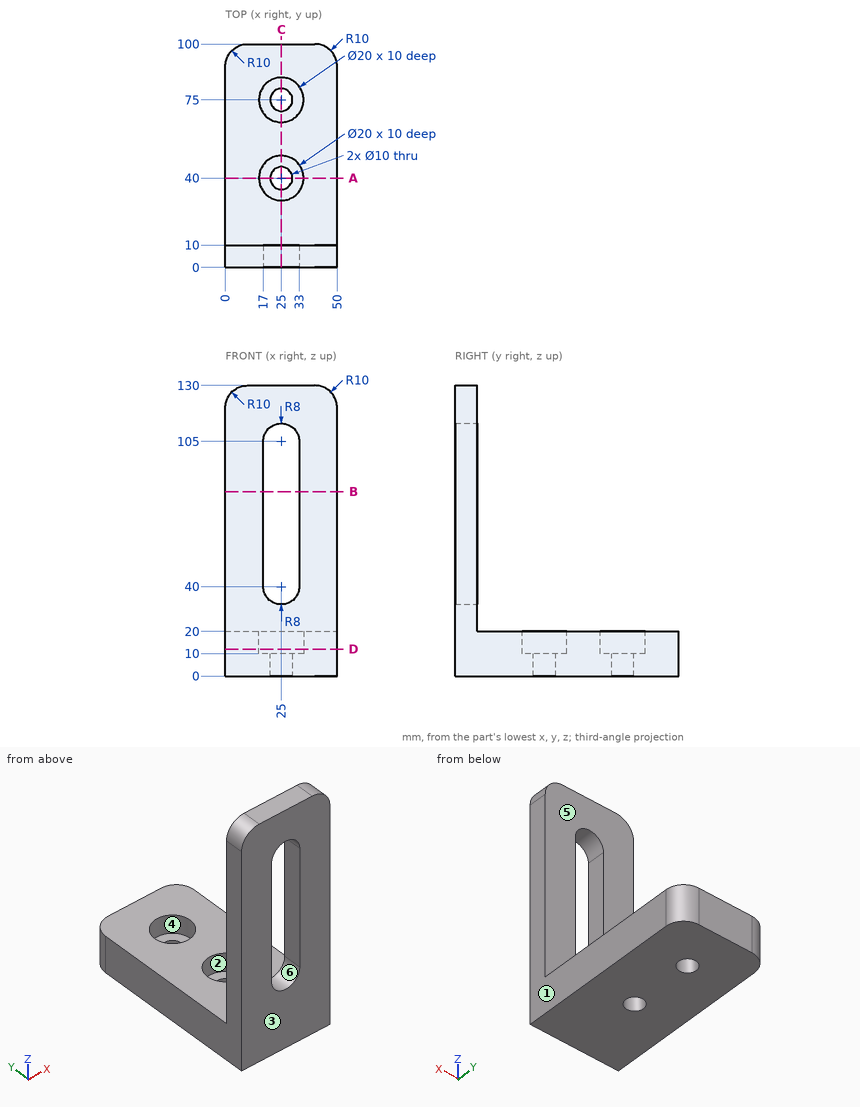
Can you work these out from the drawing? Everything is in mm from the part's minimum corner. A direction names the side the tool comes from. Coordinates: 2 decimals unless noted, no trailing zeros. Loops run counter-clockwise (first coordinate to the right, second up) from the corner with the lowest first, then second, coordinate; pieces in that order, holes last. Notation, with made-up numbers: (75, -32.5) - (91, -32.5) arc R16 cw to (91, -21.5) - close; hole circle Ø5 at (86, 24.5). An arc over 180 degrees is marked (long way). Use a Markdown table: item, result.
Item 1: I want a section at D-D on z = 12. Please give me the cut outline in (x, y), and give its area (3 significant figures).
Numbers:
| item | result |
|---|---|
| outline | (0, 0) - (50, 0) - (50, 90) arc R10 ccw to (40, 100) - (10, 100) arc R10 ccw to (0, 90) - close; hole circle Ø20 at (25, 40); hole circle Ø20 at (25, 75) |
| area | 4,330 mm2 |
Item 2: I want a section at B-B on z = 82.5. Please give me the cut outline in (x, y), and give its area (3 significant figures).
Numbers:
| item | result |
|---|---|
| outline | (0, 0) - (17, 0) - (17, 10) - (0, 10) - close; (33, 0) - (50, 0) - (50, 10) - (33, 10) - close |
| area | 340 mm2 |
Item 3: I want a section at C-C on x = 25. Please give me the cut outline in (y, z).
Numbers:
| item | result |
|---|---|
| outline | (0, 0) - (35, 0) - (35, 10) - (30, 10) - (30, 20) - (10, 20) - (10, 32) - (0, 32) - close; (0, 113) - (10, 113) - (10, 130) - (0, 130) - close; (45, 0) - (70, 0) - (70, 10) - (65, 10) - (65, 20) - (50, 20) - (50, 10) - (45, 10) - close; (80, 0) - (100, 0) - (100, 20) - (85, 20) - (85, 10) - (80, 10) - close |
Item 4: I want a section at A-A on y = 40. Please give me the cut outline in (x, z), and give its area (3 significant figures).
Numbers:
| item | result |
|---|---|
| outline | (0, 0) - (20, 0) - (20, 10) - (15, 10) - (15, 20) - (0, 20) - close; (30, 0) - (50, 0) - (50, 20) - (35, 20) - (35, 10) - (30, 10) - close |
| area | 700 mm2 |
Item 5: If I drill on probe 1 along Y at (x, z) = (25, 5.5); probe 2 along Y at (x, z) = (25, 14.75); probe 3 along Z at (x, y) = (22.5, 66), over which ranges is the centre line in solid material (lowest first)? Write a range as from..to.
Numbers:
| item | result |
|---|---|
| probe 1 | y = 0..35, 45..70, 80..100 |
| probe 2 | y = 0..30, 50..65, 85..100 |
| probe 3 | z = 0..10 |
Item 6: We'd pull the mould along Y, two halves only. Please class the marked faces 1, 2 and 3: released by +Y, released by -Y, zero draft, split by the parting line, or undercut.
Numbers:
| item | result |
|---|---|
| face 1 | zero draft |
| face 2 | undercut |
| face 3 | released by -Y |
Item 7: Will these pins go through, and if not, where does the flat tip stop? pin 1 (10 mm diameter, centred on x = 25.5, z = 36.5, fed in from -Y); pin 2 (22 mm diameter, centred on x = 26, y = 71.5, fed in from +Z); pin 3 (16 mm diameter, centred on x = 26.5, y = 41, fed in from +Z); pin 4 (1.5 mm diameter, centred on x = 35, z = 24, fed in from +Y).
Numbers:
| item | result |
|---|---|
| pin 1 | stops at y = 0 |
| pin 2 | stops at z = 20 |
| pin 3 | stops at z = 10 |
| pin 4 | stops at y = 10 |
Item 8: For the marked faces 4, 5 and 6, which set-ups out of +Z, -Z, +X, -X, +Y, -Y let a thin tool reach every point of the face, with its end or its side?
Numbers:
| item | result |
|---|---|
| face 4 | +Z |
| face 5 | +Z, +X, -X, +Y |
| face 6 | +Y, -Y |
